Autodesk Inventor part; units mm, degrees
ref_plane "YZ Plane" through (0, 0, 0) normal (1, 0, 0) x (0, 1, 0)
ref_plane "XZ Plane" through (0, 0, 0) normal (0, 1, 0) x (-1, 0, 0)
ref_plane "XY Plane" through (0, 0, 0) normal (0, 0, 1) x (1, 0, 0)
sketch "Skizze1" plane through (0, 0, 0) normal (0, 0, 1) x (1, 0, 0)
  line L0 (0, 0) -> (57, 0)
  line L1 (0, 0) -> (0, 2)
  line L2 (0, 2) -> (4, 2)
  arc A0 (6.4, 0.8) -> (4, 2) centre (4, -1) ccw
  line L3 (6.4, 0.8) -> (57, 0.8)
  line L4 (57, 0.8) -> (57, 0)
  dimension "d0" = 4
  dimension "d1" = 1.6
  dimension "d2" = 3
  dimension "d3" = 4
  dimension "d4" = 57
revolve "Umdrehung1" add sketch "Skizze1" angle 360 about axis through (0, 0, 0) along (1, 0, 0)
shell "Wandung1" thickness 0.25 removed faces 1 at (0, 0.6473, -0.1595)
properties part number "rod" material "Eisen, Grau"
Build history of the part. All positions in model axes, mm. A direction names the side the tool comes from. Coordinates: 2 decimals unless noted, no trailing zeros. Write each loop counter-clockwise with the first axis right and the second up, starting at its lowest first coordinate (ties: lowest second). Pieces come first, ordered by that corner, then holes.
(1) Mould opens along Y. For faces 3 (the cylindrical face through (2.028, 1.617, -0.67)), 4 (the cylindrical face through (2, 0, -2)), 5 (the flat face through (57, 0, 0)) say: pulls with the +Y half, pulls with the -Y half, needs draft (parallel to the pull), parting line crosses it, or undercut.
(2) Pin check, flat tips, straight feed: pin 1 Ø1.5 at (x, y) = (28, -0.5) entering from +Z; pin 2 Ø0.6 at (y, z) = (0, 0) entering from -X; pin 3 Ø2 at (x, y) = (23, 1.5) entering from +Z. Stop position of each tip, or through.
(3) Drill centre lines: line 1 (Z direction, x = 0.95, y = 0); line 2 (Z direction, x = 40.5, y = 0); line 3 (X direction, y = -0.7, z = -1.15). Where is each one in solid material? Low to high.
(4) Cut at A-A on x = 7.5. List the corners of the cut face in (y, z).
(5) 3-axis set-ups, long thin cutter, end or side, ignore diameter. For faces 1 (the cylindrical face through (32.05, -0.63, -0.49)), 2 (the flat face through (56.75, 0, 0)): which of +Z, -Z, +X, -X, +Y, -Y reach the whole face in a straight line?
Working result:
1. face 3: undercut
1. face 4: parting line crosses it
1. face 5: needs draft
2. pin 1: stops at z = 0.8
2. pin 2: stops at x = 56.75
2. pin 3: stops at z = 0.62
3. line 1: z = -2 to -1.75, 1.75 to 2
3. line 2: z = -0.8 to -0.55, 0.55 to 0.8
3. line 3: x = 5.43 to 5.87
4. outline: circle Ø1.6 at (0, 0); hole circle Ø1.1 at (0, 0)
5. face 1: +X
5. face 2: -X
